For this review, take the finished solid that the model builds, in its own axes (mm). Face numbers are marked on the shaded views. Give positions to 0.01 mm unless a question says otherwise; leave off trailing zeros. Order: outer loops, then holes, each group sorted by start corner. A loop starts at its lowest first (then second) coordinate and runs counter-clockwise, first axis right, second up. Notation, with made-up numbers: (7, 32) -> (50, 32) arc R14 cw to (50, 47) -> close; hole circle Ø11 at (2, 69). An arc over 180 degrees is marked (long way). Return JSON: item names as keys, results as strings. Group by question number.
1) Add section B-B (x = 158.75). Give the boundary of the cut face in (y, z) (3 decimals).
2) The part is to be moulded in two halves that separate along X. For the marked faces 1, 2, 3 and 4, say which applies: released by +X, released by -X, zero draft, split by the parting line, or undercut.
3) Add section A-A (y = -14.25). Give the boundary of the cut face in (x, z) (3 decimals), then the cut area to 3 significant figures.
4) To check wall thickness, follow line 1 along Z through (x, y) = (53.5, -10.5); line 2 along X through (y, z) = (-9, 110); line 3 along Y through (x, z) = (131.5, 118). State the ranges of each line that lie inside material, in increasing order.
5) Add section C-C (z = 76.2). Give the boundary of the cut face in (x, y) (3 decimals).
6) Add section D-D (x = 231.5). Give the boundary of the cut face in (y, z), then the cut area to 3 significant figures.
7) Insertion check: P1, Ø4, axis at x = 57, z = 47.5, coming from the -Y side. The pin has a flat end and moves straight along its axis. Give the tip position at first contact, or say it passes through.
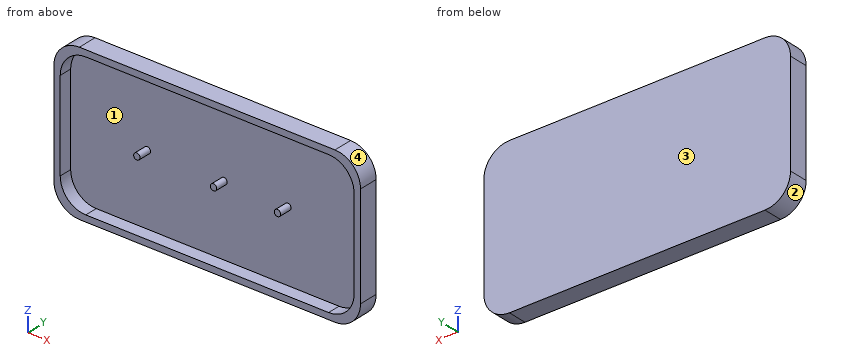
from build123d import *

# Parameters (mm, degrees)
F1_DEPTH = 19.05
F2_DEPTH = 6.35
F4_DEPTH = 12.7


with BuildPart() as f1:
    # F0 (on Front) → F1 (new body)
    with BuildSketch(Plane.XZ):
        with BuildLine():
            ThreePointArc((0, 25.4), (7.4394877579, 7.4394877579), (25.4, 0))
            Line((25.4, 0), (279.4, 0))
            ThreePointArc((279.4, 0), (297.3605122421, 7.4394877579), (304.8, 25.4))
            Line((304.8, 25.4), (304.8, 76.2))
            Line((304.8, 76.2), (298.45, 76.2))
            Line((298.45, 76.2), (298.45, 31.75))
            ThreePointArc((298.45, 31.75), (291.0105122421, 13.7894877579), (273.05, 6.35))
            Line((273.05, 6.35), (31.75, 6.35))
            ThreePointArc((31.75, 6.35), (13.7894877579, 13.7894877579), (6.35, 31.75))
            Line((6.35, 31.75), (6.35, 76.2))
            Line((6.35, 76.2), (0, 76.2))
            Line((0, 76.2), (0, 25.4))
        make_face()
        with BuildLine():
            Line((0, 127), (0, 76.2))
            Line((0, 76.2), (6.35, 76.2))
            Line((6.35, 76.2), (6.35, 120.65))
            ThreePointArc((6.35, 120.65), (13.7894877579, 138.6105122421), (31.75, 146.05))
            Line((31.75, 146.05), (273.05, 146.05))
            ThreePointArc((273.05, 146.05), (291.0105122421, 138.6105122421), (298.45, 120.65))
            Line((298.45, 120.65), (298.45, 76.2))
            Line((298.45, 76.2), (304.8, 76.2))
            Line((304.8, 76.2), (304.8, 127))
            ThreePointArc((304.8, 127), (297.3605122421, 144.9605122421), (279.4, 152.4))
            Line((279.4, 152.4), (25.4, 152.4))
            ThreePointArc((25.4, 152.4), (7.4394877579, 144.9605122421), (0, 127))
        make_face()
    extrude(amount=F1_DEPTH)

    # F0 (on Front) → F2 (join)
    with BuildSketch(Plane.XZ):
        with BuildLine():
            Line((6.35, 120.65), (6.35, 76.2))
            Line((6.35, 76.2), (298.45, 76.2))
            Line((298.45, 76.2), (298.45, 120.65))
            ThreePointArc((298.45, 120.65), (291.0105122421, 138.6105122421), (273.05, 146.05))
            Line((273.05, 146.05), (31.75, 146.05))
            ThreePointArc((31.75, 146.05), (13.7894877579, 138.6105122421), (6.35, 120.65))
        make_face()
        with BuildLine():
            Line((298.45, 76.2), (6.35, 76.2))
            Line((6.35, 76.2), (6.35, 31.75))
            ThreePointArc((6.35, 31.75), (13.7894877579, 13.7894877579), (31.75, 6.35))
            Line((31.75, 6.35), (273.05, 6.35))
            ThreePointArc((273.05, 6.35), (291.0105122421, 13.7894877579), (298.45, 31.75))
            Line((298.45, 31.75), (298.45, 76.2))
        make_face()
    extrude(amount=F2_DEPTH)

    # F3 (on face) → F4 (join)
    with BuildSketch(Plane.XZ.offset(6.35)):
        with BuildLine():
            Line((79.375, 76.2), (85.725, 76.2))
            ThreePointArc((85.725, 76.2), (82.55, 79.375), (79.375, 76.2))
        make_face()
        with BuildLine():
            ThreePointArc((79.375, 76.2), (82.55, 73.025), (85.725, 76.2))
            Line((85.725, 76.2), (79.375, 76.2))
        make_face()
        with BuildLine():
            ThreePointArc((155.575, 76.2), (158.75, 73.025), (161.925, 76.2))
            Line((161.925, 76.2), (155.575, 76.2))
        make_face()
        with BuildLine():
            Line((155.575, 76.2), (161.925, 76.2))
            ThreePointArc((161.925, 76.2), (158.75, 79.375), (155.575, 76.2))
        make_face()
        with BuildLine():
            ThreePointArc((219.075, 76.2), (222.25, 73.025), (225.425, 76.2))
            Line((225.425, 76.2), (219.075, 76.2))
        make_face()
        with BuildLine():
            Line((219.075, 76.2), (225.425, 76.2))
            ThreePointArc((225.425, 76.2), (222.25, 79.375), (219.075, 76.2))
        make_face()
    extrude(amount=F4_DEPTH)


solid = f1.part
Evaluation:
{
 "1": {"outline": "(-19.05, 0) -> (0, 0) -> (0, 152.4) -> (-19.05, 152.4) -> (-19.05, 146.05) -> (-6.35, 146.05) -> (-6.35, 79.375) -> (-19.05, 79.375) -> (-19.05, 73.025) -> (-6.35, 73.025) -> (-6.35, 6.35) -> (-19.05, 6.35) -> close"},
 "2": {"face 1": "undercut", "face 2": "released by -X", "face 3": "zero draft", "face 4": "released by +X"},
 "3": {"outline": "(0, 25.4) arc R25.4 ccw to (25.4, 0) -> (279.4, 0) arc R25.4 ccw to (304.8, 25.4) -> (304.8, 127) arc R25.4 ccw to (279.4, 152.4) -> (25.4, 152.4) arc R25.4 ccw to (0, 127) -> close; circle Ø6.35 at (82.55, 76.2); circle Ø6.35 at (158.75, 76.2); circle Ø6.35 at (222.25, 76.2); hole (6.35, 31.75) arc R25.4 ccw to (31.75, 6.35) -> (273.05, 6.35) arc R25.4 ccw to (298.45, 31.75) -> (298.45, 120.65) arc R25.4 ccw to (273.05, 146.05) -> (31.75, 146.05) arc R25.4 ccw to (6.35, 120.65) -> close", "area": "5,740 mm^2"},
 "4": {"line 1": "0 to 6.35, 146.05 to 152.4", "line 2": "0 to 6.35, 298.45 to 304.8", "line 3": "-6.35 to 0"},
 "5": {"outline": "(0, -19.05) -> (6.35, -19.05) -> (6.35, -6.35) -> (79.375, -6.35) -> (79.375, -19.05) -> (85.725, -19.05) -> (85.725, -6.35) -> (155.575, -6.35) -> (155.575, -19.05) -> (161.925, -19.05) -> (161.925, -6.35) -> (219.075, -6.35) -> (219.075, -19.05) -> (225.425, -19.05) -> (225.425, -6.35) -> (298.45, -6.35) -> (298.45, -19.05) -> (304.8, -19.05) -> (304.8, 0) -> (0, 0) -> close"},
 "6": {"outline": "(-19.05, 0) -> (0, 0) -> (0, 152.4) -> (-19.05, 152.4) -> (-19.05, 146.05) -> (-6.35, 146.05) -> (-6.35, 6.35) -> (-19.05, 6.35) -> close", "area": "1,130 mm^2"},
 "7": {"P1": "y = -6.35"}
}
